```python
from build123d import *

# Parameters (mm, degrees)
MODEL_R                 = 8
MODEL_R_2               = 6
SALIENTE_EXTRUIR1_DEPTH = 3


with BuildPart() as part:
    # Model → Saliente-Extruir1 (new body)
    with BuildSketch(Plane.XY):
        with BuildLine():
            Line((-29.638958592, -8.6229578), (5.361041408, -8.6229578))
            ThreePointArc((5.361041408, -8.6229578), (8.177920898, -7.651090282), (10.361041408, -5.6229578))
            Line((10.361041408, -5.6229578), (10.361041408, 5.3770422))
            ThreePointArc((10.361041408, 5.3770422), (10.653934627, 6.084148982), (11.361041408, 6.3770422))
            Line((11.361041408, 6.3770422), (14.361041408, 6.3770422))
            ThreePointArc((14.361041408, 6.3770422), (15.068148189, 6.084148982), (15.361041408, 5.3770422))
            Line((15.361041408, 5.3770422), (15.361041408, -12.6229578))
            ThreePointArc((15.361041408, -12.6229578), (15.653934627, -13.330064581), (16.361041408, -13.6229578))
            Line((16.361041408, -13.6229578), (38.295238995, -13.613518735))
            Line((38.295238995, -13.613518735), (70.582767323, -13.6229578))
            ThreePointArc((70.582767323, -13.6229578), (71.289874104, -13.330064581), (71.582767323, -12.6229578))
            Line((71.582767323, -12.6229578), (71.582767323, -4.6229578))
            ThreePointArc((71.582767323, -4.6229578), (71.875660542, -3.915851018), (72.582767323, -3.6229578))
            Line((72.582767323, -3.6229578), (94.361041408, -3.6229578))
            ThreePointArc((94.361041408, -3.6229578), (95.068148189, -3.330064581), (95.361041408, -2.6229578))
            Line((95.361041408, -2.6229578), (95.361041408, 7.540653568))
            Line((95.361041408, 7.540653568), (91.361041408, 7.540653568))
            Line((91.361041408, 7.540653568), (91.361041408, 10.540653568))
            Line((91.361041408, 10.540653568), (95.361041408, 10.540653568))
            Line((95.361041408, 10.540653568), (95.361041408, 13.540653568))
            ThreePointArc((95.361041408, 13.540653568), (95.068148189, 14.247760349), (94.361041408, 14.540653568))
            Line((94.361041408, 14.540653568), (72.361041408, 14.540653568))
            ThreePointArc((72.361041408, 14.540653568), (71.653934627, 14.833546787), (71.361041408, 15.540653568))
            Line((71.361041408, 15.540653568), (71.361041408, 23.540653568))
            ThreePointArc((71.361041408, 23.540653568), (71.653934627, 24.247760349), (72.361041408, 24.540653568))
            Line((72.361041408, 24.540653568), (94.361041408, 24.540653568))
            ThreePointArc((94.361041408, 24.540653568), (95.068148189, 24.833546787), (95.361041408, 25.540653568))
            Line((95.361041408, 25.540653568), (95.361041408, 28.540653568))
            Line((95.361041408, 28.540653568), (91.361041408, 28.540653568))
            Line((91.361041408, 28.540653568), (91.361041408, 31.540653568))
            Line((91.361041408, 31.540653568), (95.361041408, 31.540653568))
            Line((95.361041408, 31.540653568), (95.361041408, 41.704264936))
            ThreePointArc((95.361041408, 41.704264936), (95.068148189, 42.411371717), (94.361041408, 42.704264936))
            Line((94.361041408, 42.704264936), (72.361041408, 42.704264936))
            ThreePointArc((72.361041408, 42.704264936), (71.653934627, 42.997158154), (71.361041408, 43.704264936))
            Line((71.361041408, 43.704264936), (71.361041408, 51.704264936))
            ThreePointArc((71.361041408, 51.704264936), (71.068148189, 52.411371717), (70.361041408, 52.704264936))
            Line((70.361041408, 52.704264936), (45.361041408, 52.704264936))
            Line((45.361041408, 52.704264936), (16.361041408, 52.704264936))
            ThreePointArc((16.361041408, 52.704264936), (15.653934627, 52.411371717), (15.361041408, 51.704264936))
            Line((15.361041408, 51.704264936), (15.361041408, 33.704264936))
            ThreePointArc((15.361041408, 33.704264936), (15.068148189, 32.997158154), (14.361041408, 32.704264936))
            Line((14.361041408, 32.704264936), (11.361041408, 32.704264936))
            ThreePointArc((11.361041408, 32.704264936), (10.653934627, 32.997158154), (10.361041408, 33.704264936))
            Line((10.361041408, 33.704264936), (10.361041408, 44.704264936))
            ThreePointArc((10.361041408, 44.704264936), (8.177920898, 46.732397418), (5.361041408, 47.704264936))
            Line((5.361041408, 47.704264936), (-29.638958592, 47.704264936))
            ThreePointArc((-29.638958592, 47.704264936), (-41.789163023, 45.985500923), (-52.638958592, 40.252826715))
            ThreePointArc((-52.638958592, 40.252826715), (-48.16886463, 38.892993283), (-43.6500909, 37.704897764))
            ThreePointArc((-43.6500909, 37.704897764), (-42.942984119, 37.412004546), (-42.6500909, 36.704897764))
            Line((-42.6500909, 36.704897764), (-42.638958592, 2.3770422))
            ThreePointArc((-42.638958592, 2.3770422), (-42.931851811, 1.669935419), (-43.638958592, 1.3770422))
            ThreePointArc((-43.638958592, 1.3770422), (-48.146181418, 1.085711248), (-52.638958592, 0.622154798))
            ThreePointArc((-52.638958592, 0.622154798), (-41.945677107, -6.007356598), (-29.638958592, -8.6229578))
        make_face()
        with Locations((-29.587538582, 32.540969982)):
            Circle(MODEL_R, mode=Mode.SUBTRACT)
        with Locations((-10.486492238, 19.540969982)):
            Circle(MODEL_R_2, mode=Mode.SUBTRACT)
        with Locations((-29.587538582, 6.540969982)):
            Circle(MODEL_R, mode=Mode.SUBTRACT)
        Polygon((34.361041408, 35.540653568), (34.361041408, 20.040653568), (34.361041408, 3.540653568), (66.361041408, 3.540653568), (66.361041408, 35.540653568), align=None, mode=Mode.SUBTRACT)
        with BuildLine():
            Line((4.790372378, 29.338873837), (2.790372378, 29.338873837))
            ThreePointArc((2.790372378, 29.338873837), (2.083265597, 29.045980618), (1.790372378, 28.338873837))
            Line((1.790372378, 28.338873837), (1.790372378, 10.338873837))
            ThreePointArc((1.790372378, 10.338873837), (2.083265597, 9.631767056), (2.790372378, 9.338873837))
            Line((2.790372378, 9.338873837), (4.790372378, 9.338873837))
            ThreePointArc((4.790372378, 9.338873837), (5.49747916, 9.631767056), (5.790372378, 10.338873837))
            Line((5.790372378, 10.338873837), (5.790372378, 28.338873837))
            ThreePointArc((5.790372378, 28.338873837), (5.49747916, 29.045980618), (4.790372378, 29.338873837))
        make_face(mode=Mode.SUBTRACT)
    extrude(amount=SALIENTE_EXTRUIR1_DEPTH)


solid = part.part
```
Work out the finished part from the listing and answer in its coordinate system (mm). A direction names the side the tool comes from. Give positions to 0.01 mm unless a question says otherwise; leave off trailing zeros. Write each loop counter-clockwise with the first axis right and the second up, starting at its lowest first coordinate (ties: lowest second). Pieces come first, ordered by that corner, then holes. Notation, with made-up numbers: (79, -28.75) - (134, -28.75) arc R22 ccw to (134, 3.25) - close; hole circle Ø3 at (52.25, -15.75). An arc over 180 degrees is marked (long way). Use one line per item in the form item = value.
1. Consider L1, parallel to X at y = 20, z = 1.4; L2, parallel to X at y = 5.5, z = 2.4; L3, parallel to Y at x = -10.5, z = 1.25. Determine where each line is inside the solid, lowest interval first.
Filled in:
L1 = -42.64 to -16.47, -4.5 to 1.79, 5.79 to 34.36, 66.36 to 71.36
L2 = -42.64 to -37.52, -21.66 to 10.37, 15.35 to 34.36, 66.36 to 95.36
L3 = -8.62 to 13.54, 25.54 to 47.7
2. A cutting plane is placed at D-D (z = 0.6). State how many separate pieces and enclosed holes the cut face has, and give its area (3 significant figures).
Filled in:
separate_pieces = 1
enclosed_holes = 5
area = 6,120 mm^2
3. A cutting plane is placed at C-C (x = -11). Write down the section's boundary in (y, z).
Filled in:
outline = (-8.62, 0) - (13.56, 0) - (13.56, 3) - (-8.62, 3) - close; (25.52, 0) - (47.7, 0) - (47.7, 3) - (25.52, 3) - close
4. Determine the mould class of faces 5 (the face through (13, 6.377, 1)), 6 (the face through (-48.08, 1.09, 1.48)), 7 (the face through (84, 42.704, 1)) for opening direction X: released by +X, released by -X, zero draft, split by the parting line, or undercut.
Filled in:
face_5 = undercut
face_6 = released by -X
face_7 = zero draft
5. Each of these flat-tipped pins is pushed along its axis until it touches: pin 1 Ø1.5 at (x, z) = (-37, 1.5) entering from -Y; pin 2 Ø0.9 at (y, z) = (21, 2) entering from +X; pin 3 Ø0.9 at (x, z) = (-14, 2) entering from +Y. Where does it stop, or does it pass through?
Filled in:
pin_1 = -7.77
pin_2 = 71.36
pin_3 = 47.7
6. A cutting plane is placed at B-B (x = -31). Write down the section's boundary in (y, z).
Filled in:
outline = (-8.55, 0) - (-1.33, 0) - (-1.33, 3) - (-8.55, 3) - close; (14.42, 0) - (24.67, 0) - (24.67, 3) - (14.42, 3) - close; (40.42, 0) - (47.72, 0) - (47.72, 3) - (40.42, 3) - close
7. For faces 1 (the face through (10.361, 39, 1)), 2 (the face through (83, -3.623, 1)), 3 (the face through (8.142, -7.673, 1.479)), 4 (the face through (93, 28.541, 1)), determine the directions among +Z, -Z, +X, -X, +Y, -Y from which every point of the face is accessible in a straight line to the end or side of a thin tool.
Filled in:
face_1 = +Z, -Z, +Y
face_2 = +Z, -Z, +X, -Y
face_3 = +Z, -Z, -Y
face_4 = +Z, -Z, +X
8. A cutting plane is placed at A-A (x = 76). Write down the section's boundary in (y, z).
Filled in:
outline = (-3.62, 0) - (14.54, 0) - (14.54, 3) - (-3.62, 3) - close; (24.54, 0) - (42.7, 0) - (42.7, 3) - (24.54, 3) - close
